For this review, take the finished solid that the model builds, in its own axes (mm). Face numbers are marked on the shaded views. A direction names the side the tool comes from. Give positions to 0.01 mm unless a question says otherwise; leave off trailing zeros. Write each loop counter-clockwise with the first axis right and the second up, starting at its lowest first coordinate (ties: lowest second). Pieces come first, ordered by that corner, then holes.
1) For P1, Ø6, axis at y = -39.5, z = -5.5, coming from the +X side; P2, Ø6, axis at x = 8, z = -6.5, coming from the -Y side, all flat-tipped, find the tip position at first contact; note any pin that passes through.
2) We need section D-D on x = 26. Give the boundary of the cut face in (y, z).
3) Machinability: for the marked faces 1 and 2, which of the approach directions +Z, -Z, +X, -X, +Y, -Y give a long, thin tool a straight path to every point of the face, cutting with its end or side? Answer none if there is none.
4) We need section A-A on x = 10. Give the boundary of the cut face in (y, z), and give its area (3 significant figures).
5) We need section B-B on y = -92. Give the boundary of the cut face in (x, z), and give its area (3 significant figures).
6) We need section C-C on z = -16. Give the boundary of the cut face in (x, y).
7) Wall thickness on line 1 along Z through (x, y) = (33, -111); line 2 along X through (y, z) = (-42.5, 2.5); line 3 along Z through (x, y) = (15.5, -80): over which ranges is each line inside the solid? List them lowest first.
8) Draft analysis for pull direction Z (two halves, no side actions). For the marked faces 3, 4 and 5, state which applies: pulls with the +Z half, pulls with the -Z half, needs draft (parallel to the pull), parting line crosses it, or undercut.
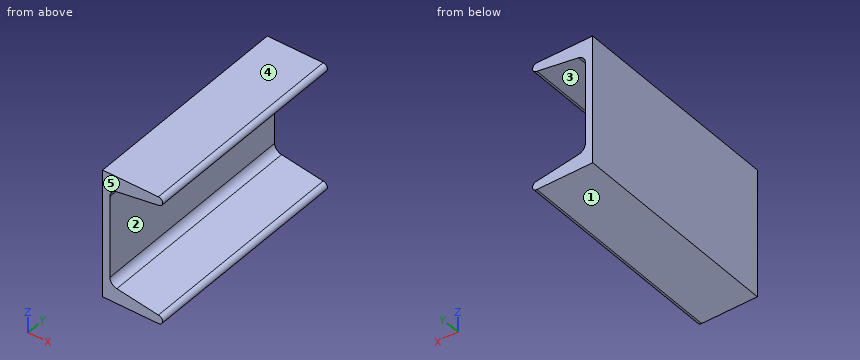
from build123d import *

# Parameters (mm, degrees)
F1_DEPTH = 127


with BuildPart() as f1:
    # F0 (on Front) → F1 (new body)
    with BuildSketch(Plane.XZ):
        with BuildLine():
            Line((4.318, 0), (4.318, 24.329558))
            ThreePointArc((4.318, 24.329558), (5.480366, 27.48029), (8.410474, 29.121229))
            Line((8.410474, 29.121229), (33.026342, 33.02))
            ThreePointArc((33.026342, 33.02), (35.566342, 35.56), (33.026342, 38.1))
            Line((33.026342, 38.1), (0, 38.1))
            Line((0, 38.1), (0, 0))
            Line((0, 0), (0, -38.1))
            Line((0, -38.1), (33.026342, -38.1))
            ThreePointArc((33.026342, -38.1), (35.566342, -35.56), (33.026342, -33.02))
            Line((33.026342, -33.02), (8.410474, -29.121229))
            ThreePointArc((8.410474, -29.121229), (5.480366, -27.48029), (4.318, -24.329558))
            Line((4.318, -24.329558), (4.318, 0))
        make_face()
    extrude(amount=F1_DEPTH)


solid = f1.part
Results list:
1. P1: stops at x = 4.32
1. P2: passes through
2. outline: (-127, -38.1) - (0, -38.1) - (0, -31.91) - (-127, -31.91) - close; (-127, 31.91) - (0, 31.91) - (0, 38.1) - (-127, 38.1) - close
3. face 1: -Z, +X, -X, +Y, -Y
3. face 2: +X, +Y, -Y
4. outline: (-127, -38.1) - (0, -38.1) - (0, -29.37) - (-127, -29.37) - close; (-127, 29.37) - (0, 29.37) - (0, 38.1) - (-127, 38.1) - close
4. area: 2,220 mm2
5. outline: (0, -38.1) - (33.03, -38.1) arc R2.54 ccw to (33.03, -33.02) - (8.41, -29.12) arc R4.85 cw to (4.32, -24.33) - (4.32, 24.33) arc R4.85 cw to (8.41, 29.12) - (33.03, 33.02) arc R2.54 ccw to (33.03, 38.1) - (0, 38.1) - close
5. area: 778 mm2
6. outline: (0, -127) - (4.32, -127) - (4.32, 0) - (0, 0) - close
7. line 1: z = -38.1 to -33.02, 33.02 to 38.1
7. line 2: x = 0 to 4.32
7. line 3: z = -38.1 to -30.24, 30.24 to 38.1
8. face 3: undercut
8. face 4: pulls with the +Z half
8. face 5: needs draft
